Source: three-view drawing plus pictorial views. Frame: mm from the lowest corner of the part. A direction names the side the tool comes from. Give positions to 0.01 mm unless a question says otherwise; leave off trailing zeros. Order: outer loops, then holes, each group sorted by start corner. A loop starts at its lowest first (then second) coordinate and runs counter-clockwise, first axis right, second up.
1) Draft query along Y for the marked faces 1, 2 and 3. Return one class per face: released by +Y, released by -Y, zero draft, split by the parting line, or undercut.
2) Section A-A, the plane z = 1.5. Give the number of separate pieces and of enclosed holes in the cut face, plus the area to 3 significant figures.
3) Material intervals for line 1 (Y direction, x = 8.25, z = 2.1); line 2 (X direction, y = 25.5, z = 1.1) (1 decimal); line 3 (X direction, y = 7.5, z = 3) (1 decimal), sorted ascending.
4) Section D-D, the plane y = 11.5. Return loops of the section in (x, z) (1 decimal).
5) Access query for the marked faces 4 and 5. Directions: +Z, -Z, +X, -X, +Y, -Y. A direction counts if a zero-diameter tool reaches every point of the face in a straight line with its end or side. Return the directions, or none.
6) First-contact query: P1, Ø3.5, axis at x = 7, y = 19, coming from the +Z side; P2, Ø1.5, axis at x = 11.5, y = 12.5, coming from the +Z side. Flat tips, straight axial feed; report the tip coordinate or a pass-through.
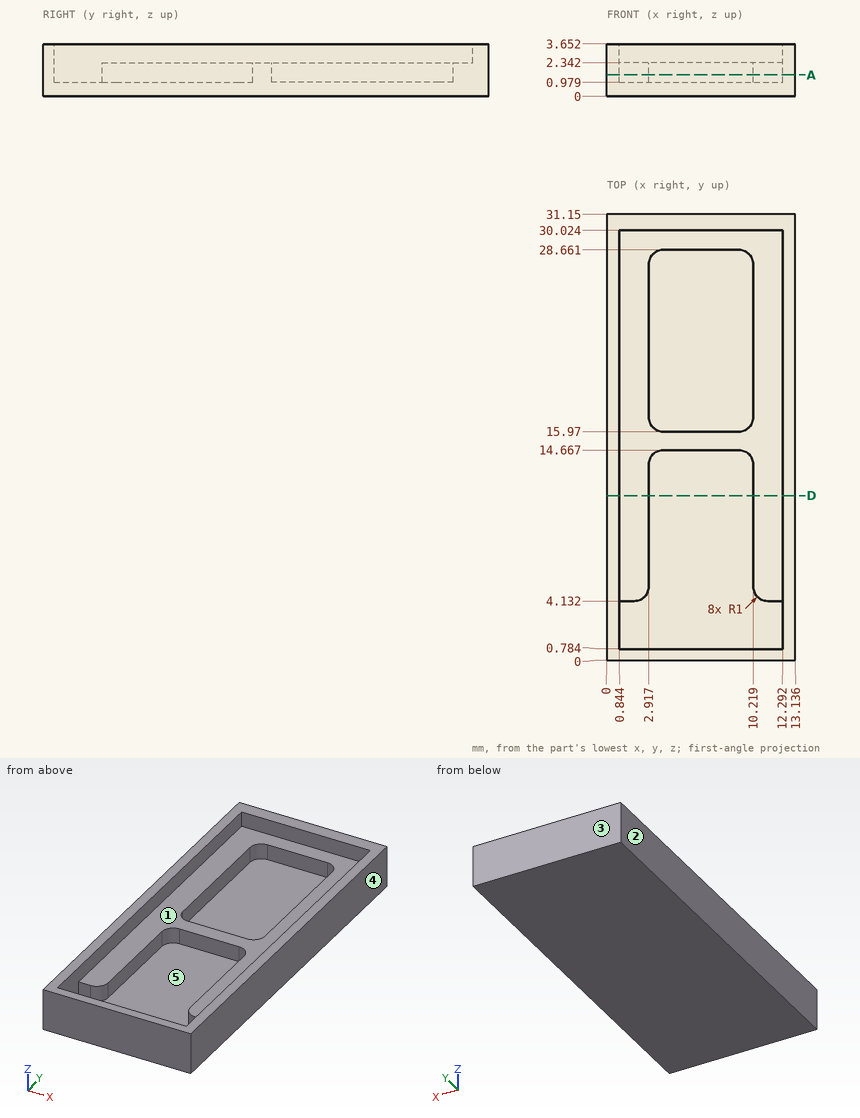
From the geometry:
1. face 1: undercut
1. face 2: zero draft
1. face 3: released by +Y
2. separate pieces: 1
2. enclosed holes: 2
2. area: 202 mm2
3. line 1: y = 0 to 0.78, 14.67 to 15.97, 28.66 to 31.15
3. line 2: x = 0 to 2.9, 10.2 to 13.1
3. line 3: x = 0 to 0.8, 12.3 to 13.1
4. outline: (0, 0) - (13.1, 0) - (13.1, 3.7) - (12.3, 3.7) - (12.3, 2.3) - (10.2, 2.3) - (10.2, 1) - (2.9, 1) - (2.9, 2.3) - (0.8, 2.3) - (0.8, 3.7) - (0, 3.7) - close
5. face 4: +Z, -Z, +X, +Y, -Y
5. face 5: +Z
6. P1: stops at z = 0.98
6. P2: stops at z = 2.34
